```python
from build123d import *

# Parameters (mm, degrees)
SKETCH1_R           = 3.3
SKETCH1_R_2         = 2.5
BOSS_EXTRUDE1_DEPTH = 3.5
SKETCH1_2_R         = 2.5
BOSS_EXTRUDE2_DEPTH = 0.6


with BuildPart() as part:
    # Sketch1 → Boss-Extrude1 (new body)
    with BuildSketch(Plane(origin=(0, 0, 0), x_dir=(1, 0, 0), z_dir=(0, 1, 0))):
        with Locations(Location((0, 0, 0), (0, 0, 270))):
            Circle(SKETCH1_R)
        with Locations(Location((0, 0, 0), (0, 0, 270))):
            Circle(SKETCH1_R_2, mode=Mode.SUBTRACT)
    extrude(amount=BOSS_EXTRUDE1_DEPTH)

    # Sketch1_2 → Boss-Extrude2 (add)
    with BuildSketch(Plane(origin=(0, 0, 0), x_dir=(1, 0, 0), z_dir=(0, 1, 0))):
        with Locations(Location((0, 0, 0), (0, 0, 270))):
            Circle(SKETCH1_2_R)
    extrude(amount=BOSS_EXTRUDE2_DEPTH)

    # Sketch2 → Revolve1 (revolve)
    with BuildSketch(Plane.XY, mode=Mode.PRIVATE) as revolve1_sk:
        Polygon((1.9, 0.6), (2.5, 0.6), (2.5, 1.2), align=None)
    revolve(revolve1_sk.sketch.rotate(Axis((0, 0, 0), (0, 1, 0)), 270), axis=Axis((0, 0, 0), (0, 1, 0)))

    # Sketch3 → Cut-Revolve2 (revolve, cut)
    with BuildSketch(Plane.XY, mode=Mode.PRIVATE) as cut_revolve2_sk:
        Polygon((3.743125207, 0), (3.743125207, 1.918181588), (2.4, 0), align=None)
    revolve(cut_revolve2_sk.sketch.rotate(Axis((0, 0, 0), (0, 1, 0)), 270), axis=Axis((0, 0, 0), (0, 1, 0)), mode=Mode.SUBTRACT)


solid = part.part
```
The listing builds one solid part. Answer for the finished solid, in the listing's coordinates (mm). Coordinates: 2 decimals unless noted, no trailing zeros. Write each loop counter-clockwise with the first axis right and the second up, starting at its lowest first coordinate (ties: lowest second). Pieces come first, ordered by that corner, then holes. Notation, with made-up numbers: (79, -15.75) - (97, -15.75) arc R29 ccw to (97, 22.25) - close; hole circle Ø11 at (51.5, 1.5). An arc over 180 degrees is marked (long way). One line per item, written item: value.
1) Find section D-D (y = 0.4). Give the vertices of the cut face in (x, z).
Geometry check:
outline: circle Ø5.36 at (0, 0)
2) For a pull along X with two mould halves and no side action, classify faces 1 (the flat face through (2, 3.5, -2)), 2 (the flat face through (0, 0.6, 0)), 3 (the cylindrical face through (-2.008, 2.377, -2.619)), 4 (the cylindrical face through (-2.44, 2.33, -0.54)) as pulls with the +X half, pulls with the -X half, needs draft (parallel to the pull), parting line crosses it, or undercut.
Geometry check:
face 1: needs draft
face 2: undercut
face 3: parting line crosses it
face 4: undercut
3) Find section A-A (z = 0). Give the vertices of the cut face in (x, y), and give its area (3 significant figures).
Geometry check:
outline: (-3.3, 1.29) - (-2.4, 0) - (2.4, 0) - (3.3, 1.29) - (3.3, 3.5) - (2.5, 3.5) - (2.5, 1.2) - (1.9, 0.6) - (-1.9, 0.6) - (-2.5, 1.2) - (-2.5, 3.5) - (-3.3, 3.5) - close
area: 7.80 mm2
4) Find section B-B (x = 0). Give the vertices of the cut face in (y, z), and give its area (3 significant figures).
Geometry check:
outline: (0, -2.4) - (1.29, -3.3) - (3.5, -3.3) - (3.5, -2.5) - (1.2, -2.5) - (0.6, -1.9) - (0.6, 1.9) - (1.2, 2.5) - (3.5, 2.5) - (3.5, 3.3) - (1.29, 3.3) - (0, 2.4) - close
area: 7.80 mm2
5) Each of these flat-tipped pins is pushed along its axis until it touches: pin 1 Ø3 at (x, z) = (-1, -1) entering from +Y; pin 2 Ø1.5 at (x, y) = (-1, 1) entering from +Z. Where does it stop, or does it pass through?
Geometry check:
pin 1: stops at y = 3.5
pin 2: stops at z = 3.29
6) Consider line 1 along X through (y, z) = (3, 0); line 2 along Z through (x, y) = (2, 0.95); line 3 along X through (y, z) = (1.95, -2). Determine where each line is inside the solid, lowest interval first. Write a range as from..to.
Geometry check:
line 1: x = -3.3..-2.5, 2.5..3.3
line 2: z = -2.32..-1.03, 1.03..2.32
line 3: x = -2.62..-1.5, 1.5..2.62
7) Find section C-C (y = 1.45). Give the vertices of the cut face in (x, z).
Geometry check:
outline: circle Ø6.6 at (0, 0); hole circle Ø5 at (0, 0)
